Source: CAD feature listing. Evaluate the final solid. Frame: model axes, mm. Face numbers are marked on the shaded views. A direction names the side the tool comes from. Give positions to 0.01 mm unless a question says otherwise; leave off trailing zeros. Loops run counter-clockwise (first coordinate to the right, second up) from the corner with the lowest first, then second, coordinate; pieces in that order, holes last. Notation, with made-up numbers: (71.5, 49.5) -> (79.5, 49.5) arc R16 ccw to (79.5, 63.5) -> close; hole circle Ø7 at (53.25, -10). An arc over 180 degrees is marked (long way). Return JSON: item names as keys, results as strings. Group by question number.
(1) Cut plane B-B on x = 9.5. Return loops of the section in (y, z).
(2) Cut plane A-A on z = 20. Give the number of separate pieces and of enclosed holes in the cut face, then the cut area to 3 significant figures.
(3) Draft query along Z for the marked faces 4, 5 and 6. Return one class per face: released by +Z, released by -Z, zero draft, split by the parting line, or undercut.
(4) Pin query (flat end, axial travel): pin 1 (12 mm diameter, centred on y = -46, z = 27.5, fed in from -X); pin 2 (15 mm diameter, centred on y = 32, z = 20, fed in from +X); pin 3 (9.5 mm diameter, centred on y = 31.5, z = 18.5, fed in from -X); pin 4 (14 mm diameter, centred on x = 45, y = -61, fed in from -Z). Return the tip coordinate at first contact, or that it passes through.
(5) Ray query, line 1 (X direction, y = -60.5, z = 11); line 2 (X direction, y = 0, z = 29); line 3 (X direction, y = -60, z = 37). Return the intervals inside material, ascending. Write a range as from..to.
(6) Cut plane C-C on y = 15. Return loops of the section in (x, z).
(7) Cut plane D-D on z = 31.5. Return loops of the section in (x, y), then the cut area to 3 significant figures.
(8) Access query for the marked faces 1, 2 and 3. Directions: +Z, -Z, +X, -X, +Y, -Y. A direction counts if a zero-diameter tool reaches every point of the face in a straight line with its end or side. Return the directions, or none.
```python
from build123d import *

# Parameters (mm, degrees)
SKETCH1_R           = 6
BOSS_EXTRUDE3_DEPTH = 40
FILLET2_R           = 10
SKETCH5_R           = 9.5
CUT_EXTRUDE1_DEPTH  = 10
SKETCH6_R           = 3
CUT_EXTRUDE2_DEPTH  = 21.5
BOSS_EXTRUDE4_START = -3
BOSS_EXTRUDE4_DEPTH = 3


with BuildPart() as part:
    # Sketch1 → Boss-Extrude3 (new body)
    with BuildSketch(Plane.XY):
        with BuildLine():
            Line((-16, -31.128764833), (-16, -61))
            ThreePointArc((-16, -61), (-11.313708499, -72.313708499), (0, -77))
            Line((0, -77), (45, -77))
            ThreePointArc((45, -77), (59.500924593, -67.761892188), (57.25671109, -50.715398245))
            Line((57.25671109, -50.715398245), (29.928255065, -18.146612597))
            ThreePointArc((29.928255065, -18.146612597), (34.869538701, -3.019150675), (32.601897088, 12.732490183))
            Line((32.601897088, 12.732490183), (20, 45))
            Line((20, 45), (1.5, 45))
            Line((1.5, 45), (1.5, 25.205406166))
            ThreePointArc((1.5, 25.205406166), (0, -25.25), (-1.5, 25.205406166))
            Line((-1.5, 25.205406166), (-1.5, 45))
            Line((-1.5, 45), (-20, 45))
            Line((-20, 45), (-32.601897088, 12.732490183))
            ThreePointArc((-32.601897088, 12.732490183), (-32.733599298, -12.389974858), (-16, -31.128764833))
        make_face()
        with Locations((0, -61)):
            Circle(SKETCH1_R, mode=Mode.SUBTRACT)
        with Locations((45, -61)):
            Circle(SKETCH1_R, mode=Mode.SUBTRACT)
    extrude(amount=BOSS_EXTRUDE3_DEPTH)

    # Fillet2
    fillet2_edges = [part.edges().sort_by_distance(p)[0] for p in [
        (-20, 45, 20),
        (20, 45, 20),
        (29.928255065, -18.146612597, 20),
        (-16, -31.128764833, 20),
    ]]
    fillet(fillet2_edges, radius=FILLET2_R)

    # Sketch5 → Cut-Extrude1 (cut)
    with BuildSketch(Plane(origin=(-20, 0, 0), x_dir=(0, 0, -1), z_dir=(1, 0, 0))):
        with Locations((-20, 32)):
            Circle(SKETCH5_R)
    cut_extrude1 = extrude(amount=-CUT_EXTRUDE1_DEPTH, mode=Mode.SUBTRACT)

    # Sketch6 → Cut-Extrude2 (cut)
    with BuildSketch(Plane.ZY.offset(20)):
        with Locations((20, 32)):
            Circle(SKETCH6_R)
    cut_extrude2 = extrude(amount=-CUT_EXTRUDE2_DEPTH, mode=Mode.SUBTRACT)

    # Mirror3: Cut-Extrude1, Cut-Extrude2 across plane
    add(cut_extrude1.mirror(Plane(origin=(0, 0, 0), x_dir=(0, 0, 1), z_dir=(1, 0, 0))), mode=Mode.SUBTRACT)
    add(cut_extrude2.mirror(Plane(origin=(0, 0, 0), x_dir=(0, 0, 1), z_dir=(1, 0, 0))), mode=Mode.SUBTRACT)

    # Sketch7 → Boss-Extrude4 (add)
    with BuildSketch(Plane.XY.offset(40).offset(BOSS_EXTRUDE4_START)):
        with BuildLine():
            ThreePointArc((22.5, 0), (-15.370426149, -16.431676725), (-1.5, 22.449944321))
            Line((-1.5, 22.449944321), (-1.5, 25.205406166))
            ThreePointArc((-1.5, 25.205406166), (-17.315996939, -18.377125727), (25.25, 0))
            ThreePointArc((25.25, 0), (18.377125727, 17.315996939), (1.5, 25.205406166))
            Line((1.5, 25.205406166), (1.5, 22.449944321))
            ThreePointArc((1.5, 22.449944321), (16.431676725, 15.370426149), (22.5, 0))
        make_face()
    extrude(amount=BOSS_EXTRUDE4_DEPTH)


solid = part.part
```
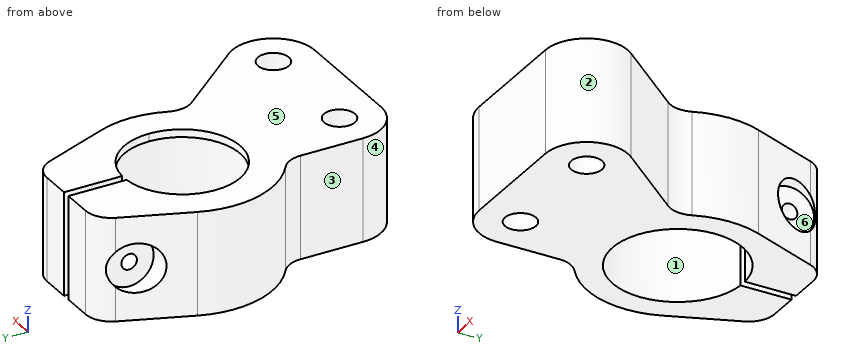
Answers:
{
 "1": {"outline": "(-77, 0) -> (-23.39, 0) -> (-23.39, 37) -> (-20.4, 37) -> (-20.4, 40) -> (-77, 40) -> close; (20.4, 37) -> (23.39, 37) -> (23.39, 0) -> (45, 0) -> (45, 40) -> (20.4, 40) -> close; hole circle Ø6 at (32, 20)"},
 "2": {"separate pieces": "3", "enclosed holes": "2", "area": "5,020 mm²"},
 "3": {"face 4": "zero draft", "face 5": "released by +Z", "face 6": "undercut"},
 "4": {"pin 1": "x = -16", "pin 2": "x = 20", "pin 3": "x = -20", "pin 4": "z = 0"},
 "5": {"line 1": "-16..-5.98, 5.98..39.02, 50.98..60.99", "line 2": "-35..-25.25, 25.25..35", "line 3": "-16..-5.92, 5.92..39.08, 50.92..60.97"},
 "6": {"outline": "(-31.72, 0) -> (-20.31, 0) -> (-20.31, 37) -> (-16.77, 37) -> (-16.77, 40) -> (-31.72, 40) -> close; (16.77, 37) -> (20.31, 37) -> (20.31, 0) -> (31.72, 0) -> (31.72, 40) -> (16.77, 40) -> close"},
 "7": {"outline": "(-32.6, 12.73) arc R35 ccw to (-20.22, -28.57) arc R10 cw to (-16, -36.73) -> (-16, -61) arc R16 ccw to (0, -77) -> (45, -77) arc R16 ccw to (57.26, -50.72) -> (34.12, -23.14) arc R10 cw to (32.5, -13) arc R35 ccw to (32.6, 12.73) -> (22.48, 38.64) arc R10 ccw to (13.17, 45) -> (1.5, 45) -> (1.5, 25.21) arc R25.25 cw (long way) to (-1.5, 25.21) -> (-1.5, 45) -> (-13.17, 45) arc R10 ccw to (-22.48, 38.64) -> close; hole circle Ø12 at (0, -61); hole circle Ø12 at (45, -61)", "area": "5,440 mm²"},
 "8": {"face 1": "-Z", "face 2": "+Z, -Z, +X", "face 3": "+Z, -Z, -X, -Y"}
}
